Part model, mm, in its own coordinate system. A direction names the side the tool comes from. Round coordinates to 2 decimals unless told otherwise and drop trailing zeros. Order: outer loops, then holes, each group sorted by start corner. A loop starts at its lowest first (then second) coordinate and runs counter-clockwise, first axis right, second up. Notation, with made-up numbers: (-38, 74.5) - (-32, 74.5) arc R5 cw to (-32, 81.5) - close; hole circle Ø6 at (-7.75, 32). An arc over 180 degrees is marked (long way). Return JSON: item names as keys, results as strings. Group by question number.
Item 1: Tool access for faces 1 (the face through (-10, 21, 17.486)), 2 (the face through (-41.94, 41.95, 4.03)), 3 (the face through (-31, 21, 23.087)), 4 (the face through (-53, 21, 17.486)): list every direction of +Z, -Z, +X, -X, +Y, -Y with a clear straight run to the whole face (end or side of a thin tool).
Item 2: Saw through at C-C on x = -53. List the corners of the cut face in (y, z), and give its area (3 significant figures).
Item 3: Drop flat-ended pins along their axis: pin 1 (8 mm diameter, centred on x = -21, y = 12, fed in from +Z); pin 2 (12 mm diameter, centred on x = -46.5, y = 36.5, fed in from -Z); pin 3 (6.5 mm diameter, centred on x = -53, y = 18.5, fed in from -Z); pin 4 (1.5 mm diameter, centred on y = 13, z = 4.5, fed in from +X). Give the stop position or say it passes through.
Item 4: Two-plate mould, pull along Y, no slides. Class faces 5 (the face through (-37.3, 21.2, 5.1)), 6 (the face through (-50.902, 32.932, 20.648)), 7 (the face through (-31, 42.951, 18)), 8 (the face through (-31, 0, 18)): released by +Y, released by -Y, zero draft, split by the parting line, or undercut.
Item 5: Saw through at A-A on z = 3. List the corners of the cut face in (x, y).
Item 6: Saw through at D-D on x = -32.5. List the corners of the cut face in (y, z), and give its area (3 significant figures).
Item 7: Probe probe 1 along X at (y, z) = (34, 20); probe 2 along Z at (x, y) = (-13.5, 20); probe 3 along X at (y, z) = (9, 4). List the from-to ranges inside material, lowest first.
```python
from build123d import *

# Parameters (mm, degrees)
SKETCH1_R           = 6.35
BOSS_EXTRUDE1_DEPTH = 42.9514
SKETCH2_R           = 11.1125
CUT_EXTRUDE1_DEPTH  = 2.032
CUT_EXTRUDE2_START  = -2.032
SKETCH3_R           = 11.1125
CUT_EXTRUDE2_DEPTH  = 2.032
SKETCH8_R           = 2.0447
CUT_EXTRUDE3_DEPTH  = 76.496791448


with BuildPart() as part:
    # Sketch1 → Boss-Extrude1 (new body)
    with BuildSketch(Plane(origin=(0, 0, 0), x_dir=(1, 0, 0), z_dir=(0, 1, 0))):
        with BuildLine():
            Line((-41.729120795, -23.848667038), (-41.729120795, -23.899467038))
            Line((-41.729120795, -23.899467038), (-56.683370795, -23.899467038))
            Line((-56.683370795, -23.899467038), (-56.683370795, -17.485967038))
            Line((-56.683370795, -17.485967038), (-48.364870795, -17.485967038))
            Line((-48.364870795, -17.485967038), (-48.364870795, 4.645738735))
            Line((-48.364870795, 4.645738735), (-40.109870795, 4.645738735))
            ThreePointArc((-40.109870795, 4.645738735), (-31.092870795, 7.850532962), (-22.075870795, 4.645738735))
            Line((-22.075870795, 4.645738735), (-13.820870795, 4.645738735))
            Line((-13.820870795, 4.645738735), (-13.820870795, -17.485967038))
            Line((-13.820870795, -17.485967038), (-5.502370795, -17.485967038))
            Line((-5.502370795, -17.485967038), (-5.502370795, -23.899467038))
            Line((-5.502370795, -23.899467038), (-20.456620795, -23.899467038))
            Line((-20.456620795, -23.899467038), (-20.456620795, -23.848667038))
            ThreePointArc((-20.456620795, -23.848667038), (-20.679805428, -23.309851671), (-21.218620795, -23.086667038))
            Line((-21.218620795, -23.086667038), (-40.967120795, -23.086667038))
            ThreePointArc((-40.967120795, -23.086667038), (-41.505936162, -23.309851671), (-41.729120795, -23.848667038))
        make_face()
        with Locations(Location((-31.092870795, -6.436967038, 0), (0, 0, 270))):
            Circle(SKETCH1_R, mode=Mode.SUBTRACT)
    extrude(amount=BOSS_EXTRUDE1_DEPTH)

    # Sketch2 → Cut-Extrude1 (cut)
    with BuildSketch(Plane(origin=(0, 42.9514, 0), x_dir=(1, 0, 0), z_dir=(0, 1, 0))):
        with Locations(Location((-31.092870795, -6.436967038, 0), (0, 0, 270))):
            Circle(SKETCH2_R)
    extrude(amount=-CUT_EXTRUDE1_DEPTH, mode=Mode.SUBTRACT)

    # Sketch3 → Cut-Extrude2 (cut)
    with BuildSketch(Plane.XZ.offset(CUT_EXTRUDE2_START)):
        with Locations(Location((-31.092870795, 6.436967038, 0), (0, 0, 90))):
            Circle(SKETCH3_R)
    extrude(amount=CUT_EXTRUDE2_DEPTH, mode=Mode.SUBTRACT)

    # Sketch8 → Cut-Extrude3 (cut, through all)
    with BuildSketch(Plane(origin=(0, 0, 17.485967038), x_dir=(-1, 0, 0), z_dir=(0, 0, -1))):
        with Locations((52.524120795, 8.7757)):
            Circle(SKETCH8_R)
        with Locations((52.524120795, 34.1757)):
            Circle(SKETCH8_R)
        with Locations((9.661620795, 8.7757)):
            Circle(SKETCH8_R)
        with Locations((9.661620795, 34.1757)):
            Circle(SKETCH8_R)
    extrude(amount=-CUT_EXTRUDE3_DEPTH, mode=Mode.SUBTRACT)


solid = part.part
```
Filled in:
{
 "1": {"face 1": "-Z, +X, +Y, -Y", "face 2": "+Y", "face 3": "+Z, +Y, -Y", "face 4": "-Z, -X, +Y, -Y"},
 "2": {"outline": "(0, 17.49) - (6.79, 17.49) - (6.79, 23.9) - (0, 23.9) - close; (10.76, 17.49) - (32.19, 17.49) - (32.19, 23.9) - (10.76, 23.9) - close; (36.16, 17.49) - (42.95, 17.49) - (42.95, 23.9) - (36.16, 23.9) - close", "area": "224 mm^2"},
 "3": {"pin 1": "stops at z = 23.9", "pin 2": "stops at z = -4.65", "pin 3": "stops at z = 17.49", "pin 4": "stops at x = -13.82"},
 "4": {"face 5": "zero draft", "face 6": "undercut", "face 7": "released by +Y", "face 8": "released by -Y"},
 "5": {"outline": "(-48.36, 0) - (-41.66, 0) - (-41.66, 2.03) - (-36.43, 2.03) - (-36.43, 40.92) - (-41.66, 40.92) - (-41.66, 42.95) - (-48.36, 42.95) - close; (-25.75, 2.03) - (-20.53, 2.03) - (-20.53, 0) - (-13.82, 0) - (-13.82, 42.95) - (-20.53, 42.95) - (-20.53, 40.92) - (-25.75, 40.92) - close"},
 "6": {"outline": "(0, -7.78) - (42.95, -7.78) - (42.95, -4.59) - (40.92, -4.59) - (40.92, 0.24) - (2.03, 0.24) - (2.03, -4.59) - (0, -4.59) - close; (0, 17.46) - (2.03, 17.46) - (2.03, 12.63) - (40.92, 12.63) - (40.92, 17.46) - (42.95, 17.46) - (42.95, 23.09) - (0, 23.09) - close", "area": "755 mm^2"},
 "7": {"probe 1": "x = -56.68 to -54.56, -50.49 to -11.7, -7.62 to -5.5", "probe 2": "z = 17.49 to 23.9", "probe 3": "x = -48.36 to -36.96, -25.23 to -13.82"}
}
